Autodesk Inventor part; units mm, degrees
ref_plane "YZ Plane" through (0, 0, 0) normal (1, 0, 0) x (0, 1, 0)
ref_plane "XZ Plane" through (0, 0, 0) normal (0, 1, 0) x (-1, 0, 0)
ref_plane "XY Plane" through (0, 0, 0) normal (0, 0, 1) x (1, 0, 0)
sketch "Skizze1" plane through (0, 0, 0) normal (0, 1, 0) x (-1, 0, 0)
  line L0 (144.9597, 31.6532) -> (-5.0403, 31.6532)
  line L1 (-5.0403, 31.6532) -> (-5.0403, -118.3468)
  line L2 (-5.0403, -118.3468) -> (144.9597, -118.3468)
  line L3 (144.9597, -118.3468) -> (144.9597, 31.6532)
  line L4 (144.9597, 31.6532) -> (-5.0403, -118.3468) construction
  line L5 (-5.0403, 31.6532) -> (144.9597, -118.3468) construction
  point P0 (0, 0)
  point P1 (69.9597, -43.3468)
  dimension "d0" = 150
  dimension "d1" = 150
extrude "Extrusion1" add sketch "Skizze1" along normal blind 5
sketch "Skizze2" plane through (0, 5, 0) normal (0, 1, 0) x (1, 0, 0)
  circle A0 centre (-134.9597, -21.6532) radius 2.5
  circle A1 centre (-134.9597, 108.3468) radius 2.5
  circle A2 centre (-4.9597, -21.6532) radius 2.5
  circle A3 centre (-4.9597, 108.3468) radius 2.5
  line L0 (-144.9597, 118.3468) -> (-144.9597, -31.6532)
  line L1 (-144.9597, -31.6532) -> (5.0403, -31.6532)
  line L2 (5.0403, 118.3468) -> (-144.9597, 118.3468)
  line L3 (5.0403, -31.6532) -> (5.0403, 118.3468)
  point P0 (0, 0)
  dimension "d4" = 5
  dimension "d5" = 5
  dimension "d6" = 5
  dimension "d7" = 5
  dimension "d8" = 10
  dimension "d9" = 10
  dimension "d15" = 10
  dimension "d16" = 10
  dimension "d17" = 10
  dimension "d18" = 10
  dimension "d19" = 10
  dimension "d20" = 10
hole "Bohrung1" at (-134.9597, 5, 21.6532) at (-134.9597, 5, -108.3468) at (-4.9597, 5, -108.3468) at (-4.9597, 5, 21.6532) direction (0, -1, 0) diameter 4.978 depth 19.05 tip angle 118
properties part number "Grundplatte"
Source: CAD feature listing. Evaluate the final solid. Frame: model axes, mm. Round coordinates to 2 decimals unless told otherwise and drop trailing zeros. Order: outer loops, then holes, each group sorted by start corner. A loop starts at its lowest first (then second) coordinate and runs counter-clockwise, first axis right, second up. Notation, with made-up numbers: (-6.5, 63.5) - (15.5, 63.5) arc R36 ccw to (15.5, 101.5) - close; hole circle Ø2 at (18.25, -10). An arc over 180 degrees is marked (long way). Use a Markdown table: item, result. Add a question column.
1. Mould query, pull axis X, two halves, no side actions, for faces 1 (the cylindrical face through (-137.428, 2.465, -108.671)), 2 (the flat face through (5.04, 2, -42)), 3 (the flat face through (-69, 5, -42)). Classes: +X half, -X half, draft (parallel to the pull), parting line (faces both ways), or undercut.
2. Section query A-A (z = -108). Return the cut outline in (x, y), then the cut area to 3 significant figures.
3. Line query: probe 1 along X at (y, z) = (3.3, 22); probe 2 along X at (y, z) = (2.05, 19.5). Output: solid intervals per line, ascending.
Derived:
| question | item | result |
|---|---|---|
| 1 | face 1 | undercut |
| 1 | face 2 | +X half |
| 1 | face 3 | draft |
| 2 | outline | (-144.96, 0) - (-137.42, 0) - (-137.42, 5) - (-144.96, 5) - close; (-132.49, 0) - (-7.42, 0) - (-7.42, 5) - (-132.49, 5) - close; (-2.49, 0) - (5.04, 0) - (5.04, 5) - (-2.49, 5) - close |
| 2 | area | 701 mm2 |
| 3 | probe 1 | -144.96 to -137.42, -132.49 to -7.42, -2.49 to 5.04 |
| 3 | probe 2 | -144.96 to -136.21, -133.71 to -6.21, -3.71 to 5.04 |
